Verification items for this drawing (mm, ordinates from the low corner). A direction names the side the tool comes from. Coordinates: 2 decimals unless noted, no trailing zeros. Write each loop counter-clockwise with the first axis right and the second up, starting at its lowest first coordinate (ties: lowest second). Pieces come first, ordered by that corner, then holes. Notation, with made-up numbers: (-19, 59) -> (25, 59) arc R20 ccw to (25, 98) -> close; hole circle Ø7 at (41.25, 47.5). An arc over 180 degrees is marked (long way). One line per question, with ' | ' between items.
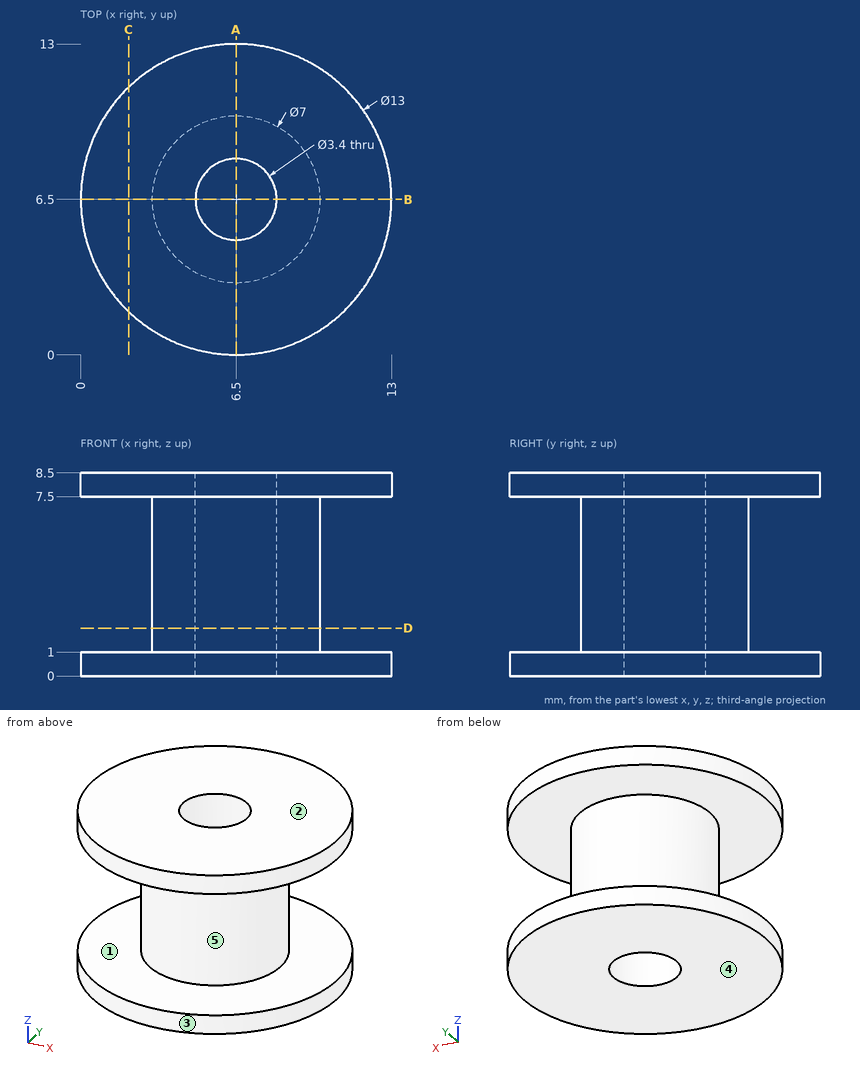
(1) Depth check by flat-ended pin: P1, Ø2, axis at y = 7.5, z = 1.5, coming from the -X side; P2, Ø3, axis at x = 3.5, z = 1, coming from the +Y side; P3, Ø5.5, axis at x = 6.5, y = 6.5, coming from the +Z side. Enter the tip coordinate at first touch or a pass-through.
Answers below:
P1: stops at x = 0 | P2: stops at y = 12.82 | P3: stops at z = 8.5
(2) Material ranges on line 1 (Z direction, x = 9.5, y = 2.75); line 2 (X direction, y = 6.5, z = 5.5), recorded low to high.
Answers below:
line 1: z = 0 to 1, 7.5 to 8.5 | line 2: x = 3 to 4.8, 8.2 to 10
(3) Tool access check on the marked faces 4 and 5. Record the directions out of +Z, -Z, +X, -X, +Y, -Y that give a thin tool (end or side, any length) a straight path to the whole face; none if there is none.
Answers below:
face 4: -Z, +X, -X, +Y, -Y | face 5: none
(4) Cross-section at A-A (x = 6.5). Record the cut outline in (y, z).
Answers below:
outline: (0, 0) -> (4.8, 0) -> (4.8, 8.5) -> (0, 8.5) -> (0, 7.5) -> (3, 7.5) -> (3, 1) -> (0, 1) -> close; (8.2, 0) -> (13, 0) -> (13, 1) -> (10, 1) -> (10, 7.5) -> (13, 7.5) -> (13, 8.5) -> (8.2, 8.5) -> close
(5) Draft check along Z on the marked faces 1, 2 and 3. Enter one of: pulls with the +Z half, pulls with the -Z half, needs draft (parallel to the pull), parting line crosses it, or undercut.
Answers below:
face 1: undercut | face 2: pulls with the +Z half | face 3: needs draft
(6) Cross-section at D-D (z = 2). Record the cut outline in (x, y).
Answers below:
outline: circle Ø7 at (6.5, 6.5); hole circle Ø3.4 at (6.5, 6.5)
(7) Cross-section at C-C (x = 2). Record the cut outline in (y, z), plus the area to 3 significant figures.
Answers below:
outline: (1.81, 0) -> (11.19, 0) -> (11.19, 1) -> (1.81, 1) -> close; (1.81, 7.5) -> (11.19, 7.5) -> (11.19, 8.5) -> (1.81, 8.5) -> close | area: 18.8 mm²
